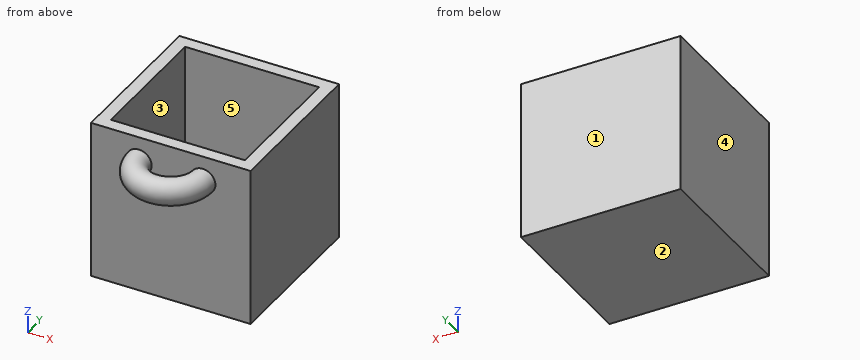
from build123d import *

# Parameters (mm, degrees)
BOX001_W     = 21
BOX001_H     = 21
BOX001_DEPTH = 24
TORUS_R      = 2
BOX_W        = 25
BOX_H        = 25
BOX_DEPTH    = 25


with BuildPart() as cube001:
    # Box001 → Box001 (new body)
    with BuildSketch(Plane(origin=(2, 2, 2), x_dir=(1, 0, 0), z_dir=(0, 0, 1))):
        with Locations((10.5, 10.5)):
            Rectangle(BOX001_W, BOX001_H)
    extrude(amount=BOX001_DEPTH)


with BuildPart() as torus:
    # Torus → Torus (revolve)
    with BuildSketch(Plane(origin=(12.5, 0, 21), x_dir=(1, 0, 0), z_dir=(0, -1, 0))):
        with Locations((5, 0)):
            Circle(TORUS_R)
    revolve(axis=Axis((12.5, 0, 21), (0, 0, 1)))


with BuildPart() as cut:
    # Box → Box (new body)
    with BuildSketch(Plane.XY):
        with Locations((12.5, 12.5)):
            Rectangle(BOX_W, BOX_H)
    extrude(amount=BOX_DEPTH)

    # Fusion: union Torus
    add(torus.part)

    # Cut: cut Cube001
    add(cube001.part, mode=Mode.SUBTRACT)


solid = cut.part
Geometry: final body of the model. Coordinates: model frame, mm. Face numbers are marked on the shaded views. A direction names the side the tool comes from. Give positions to 0.01 mm unless a question says otherwise; leave off trailing zeros. Loops run counter-clockwise (first coordinate to the right, second up) from the corner with the lowest first, then second, coordinate; pieces in that order, holes last. Notation, with made-up numbers: (60.25, 81.5) -> (107.25, 81.5) arc R27 ccw to (107.25, 101.5) -> close; hole circle Ø8 at (-34, -22). An arc over 180 degrees is marked (long way). Put each result on its own line as item: value.
1. Pull-direction query (Y, two-part tool) for the marked faces 1, 2 and 3; classes: released by +Y, released by -Y, zero draft, split by the parting line, or undercut.
Taken from the geometry:
face 1: released by +Y
face 2: zero draft
face 3: undercut
2. Ray query, line 1 along X through (y, z) = (6, 4.5); line 2 along Y through (x, z) = (13.5, 21.25). Return the intervals inside material, ascending. Write a range as [from, to].
Taken from the geometry:
line 1: x = [0, 2], [23, 25]
line 2: y = [-6.91, -2.85], [0, 2], [23, 25]
3. Cut plane B-B (z = 20.5). Return the cut outline in (x, y), plus the area to 3 significant figures.
Taken from the geometry:
outline: (0, 0) -> (5.56, 0) arc R6.94 ccw to (19.44, 0) -> (25, 0) -> (25, 25) -> (0, 25) -> close; hole (2, 2) -> (23, 2) -> (23, 23) -> (2, 23) -> close; hole (9.44, 0) arc R3.06 ccw to (15.56, 0) -> close
area: 245 mm2
4. Pin query (flat end, axial travel): P1, Ø10.5, axis at x = 14, z = 10.5, coming from the -Y side; P2, Ø1.5, axis at x = 10.5, y = 16, coming from the -Z side; P3, Ø3, axis at x = 6.5, y = 17.5, coming from the +Z side; P4, Ø1, axis at x = 11.5, y = -3, coming from the +Z side. Return the tip coordinate at first contact, or that it passes through.
Taken from the geometry:
P1: stops at y = 0
P2: stops at z = 0
P3: stops at z = 2
P4: stops at z = 22.49
5. Cut plane A-A (z = 7.5). Return the cut outline in (x, y).
Taken from the geometry:
outline: (0, 0) -> (25, 0) -> (25, 25) -> (0, 25) -> close; hole (2, 2) -> (23, 2) -> (23, 23) -> (2, 23) -> close
6. Set-up query: the marked faces 4 and 5. Return all of +Z, -Z, +X, -X, +Y, -Y with unobstructed straight access to the full face (end or side cutting, diameter ignored); none if empty.
Taken from the geometry:
face 4: +Z, -Z, -X, +Y, -Y
face 5: +Z
7. Cut plane C-C (y = 22). Return the cut outline in (x, z), plus the area to 3 significant figures.
Taken from the geometry:
outline: (0, 0) -> (25, 0) -> (25, 25) -> (23, 25) -> (23, 2) -> (2, 2) -> (2, 25) -> (0, 25) -> close
area: 142 mm2
